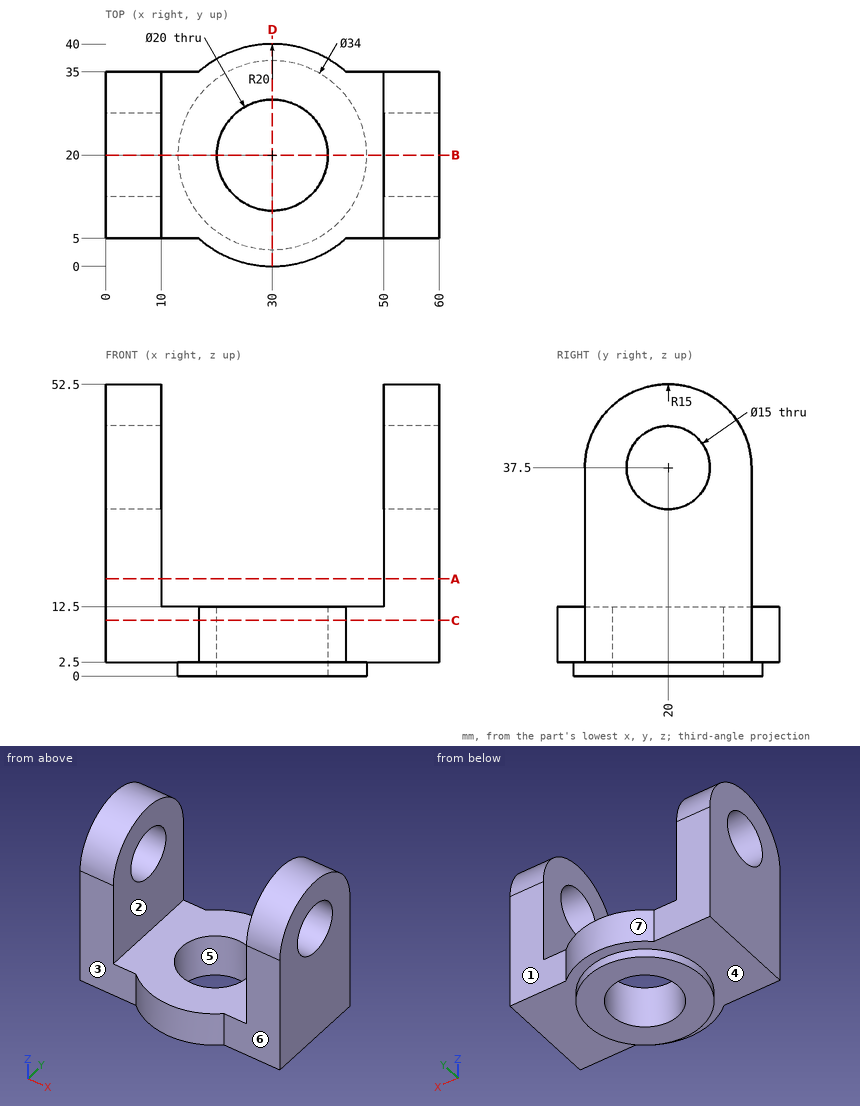
The drawing under review shows one solid part. Ordinate dimensions are in mm from its lowest x, y, z. A direction names the side the tool comes from. Coordinates: 2 decimals unless noted, no trailing zeros. Order: outer loops, then holes, each group sorted by start corner. A loop starts at its lowest first (then second) coordinate and runs counter-clockwise, first axis right, second up. Notation, with made-up numbers: (-18.5, 55) -> (29.5, 55) arc R24 ccw to (29.5, 89) -> close; hole circle Ø8 at (59, 16). An arc over 180 degrees is marked (long way). Use CSV: the item, a comma, the result in double quotes. Start each with the question number.
Item 1: We need section C-C, the plane z = 10. Give the boundary of the cut face in (x, y).
Item 2: We need section A-A, the plane z = 17.5. Give the boundary of the cut face in (x, y).
Item 3: We need section D-D, the plane x = 30. Give the boundary of the cut face in (y, z).
Item 4: Wall thickness on probe 1 along Y at (x, z) = (30, 8.5); probe 2 along X at (y, z) = (17.5, 19); probe 3 along Z at (x, y) = (7, 20): over which ranges is each line inside the solid? List them lowest first.
Item 5: Draft analysis for pull direction X (two halves, no side actions). For the marked faces 5, 6 and 7, state which applies: pulls with the +X half, pulls with the -X half, needs draft (parallel to the pull), parting line crosses it, or undercut.
Item 6: Insertion check: pin 1 (8 mm diameter, centred on x = 47.5, z = 29.5, fed in from -Y); pin 2 (8 mm diameter, centred on x = 52.5, y = 32.5, fed in from -Z); pin 3 (18.5 mm diameter, centred on x = 48, z = 18.5, fed in from -Y). Each pin has a flat end and moves straight along its axis. Give the tip position at first contact, or say it passes through.
Item 7: We need section B-B, the plane y = 20. Give the boundary of the cut face in (x, z), then the cut area to 3 significant figures.
Item 8: For the marked faces 1, 2, 3 and 4, list the 3-axis set-ups (+Z, -Z, +X, -X, +Y, -Y) from which the entire face can be reached by the end or side of a thin tool; tool diameter is ignored.
Derived:
1,outline,"(0, 5) -> (16.77, 5) arc R20 ccw to (43.23, 5) -> (60, 5) -> (60, 35) -> (43.23, 35) arc R20 ccw to (16.77, 35) -> (0, 35) -> close; hole circle Ø20 at (30, 20)"
2,outline,"(0, 5) -> (10, 5) -> (10, 35) -> (0, 35) -> close; (50, 5) -> (60, 5) -> (60, 35) -> (50, 35) -> close"
3,outline,"(0, 2.5) -> (3, 2.5) -> (3, 0) -> (10, 0) -> (10, 12.5) -> (0, 12.5) -> close; (30, 0) -> (37, 0) -> (37, 2.5) -> (40, 2.5) -> (40, 12.5) -> (30, 12.5) -> close"
4,probe 1,"y = 0 to 10, 30 to 40"
4,probe 2,"x = 0 to 10, 50 to 60"
4,probe 3,"z = 2.5 to 30, 45 to 52.5"
5,face 5,"undercut"
5,face 6,"needs draft"
5,face 7,"parting line crosses it"
6,pin 1,"stops at y = 5"
6,pin 2,"stops at z = 2.5"
6,pin 3,"stops at y = 3.27"
7,outline,"(0, 2.5) -> (13, 2.5) -> (13, 0) -> (20, 0) -> (20, 12.5) -> (10, 12.5) -> (10, 30) -> (0, 30) -> close; (0, 45) -> (10, 45) -> (10, 52.5) -> (0, 52.5) -> close; (40, 0) -> (47, 0) -> (47, 2.5) -> (60, 2.5) -> (60, 30) -> (50, 30) -> (50, 12.5) -> (40, 12.5) -> close; (50, 45) -> (60, 45) -> (60, 52.5) -> (50, 52.5) -> close"
7,area,"935 mm^2"
8,face 1,"+Z, -Z, +X, +Y"
8,face 2,"+Z, +Y, -Y"
8,face 3,"+Z, -Z, -X, -Y"
8,face 4,"-Z"
